Verification items for the finished model (mm, model axes). A direction names the side the tool comes from. Coordinates: 2 decimals unless noted, no trailing zeros. Order: outer loops, then holes, each group sorted by start corner. A loop starts at its lowest first (then second) coordinate and runs counter-clockwise, first axis right, second up. Notation, with made-up numbers: M 27,64 L 43,64 A22 cw 43,103 Z; hole C 62,48 d11. An arc over 180 degrees is marked long. Return JSON: item names as keys, results as strings.
Autodesk Inventor part; units mm, degrees
ref_plane "YZ Plane" through (0, 0, 0) normal (1, 0, 0) x (0, 1, 0)
ref_plane "XZ Plane" through (0, 0, 0) normal (0, 1, 0) x (-1, 0, 0)
ref_plane "XY Plane" through (0, 0, 0) normal (0, 0, 1) x (1, 0, 0)
sketch "Esquisse1" plane through (0, 0, 0) normal (0, 1, 0) x (-1, 0, 0)
  circle A0 centre (0, 0) radius 1.45
  circle A1 centre (0, 0) radius 4
  dimension "d0" = 8
  dimension "d1" = 2.9
extrude "Extrusion1" add sketch "Esquisse1" along normal blind 7
sketch "Esquisse2" plane through (0, 7, 0) normal (0, 1, 0) x (1, 0, 0)
  circle A0 centre (0, 0) radius 1.45
  circle A1 centre (0, 0) radius 4
  arc A2 (-2.3049, 1.5) -> (2.3049, 1.5) centre (0, 0) ccw
  line L0 (-2.3049, 1.5) -> (2.3049, 1.5)
  arc A3 (2.3049, 1.5) -> (-2.3049, 1.5) centre (0, 0) ccw construction
  dimension "d4" = 5.5
  dimension "d5" = 1.5
extrude "Extrusion2" add sketch "Esquisse2" along normal blind 8 contours A1
sketch "Esquisse3" plane through (-2.3049, 7, -1.5) normal (0, 0, 1) x (1, 0, 0)
  line L0 (4.6098, 0) -> (0, 0)
  line L1 (4.6098, 0) -> (4.6098, 8)
  line L2 (0, 8) -> (4.6098, 8)
  line L3 (1.3049, 7.2) -> (3.3049, 7.2)
  line L4 (3.3049, 7.2) -> (3.3049, 0.8)
  line L5 (3.3049, 0.8) -> (1.3049, 0.8)
  line L6 (1.3049, 0.8) -> (1.3049, 7.2)
  point P0 (2.3049, -7)
  dimension "d8" = 2
  dimension "d9" = 0.8
  dimension "d10" = 0.8
  dimension "d11" = 1.3049
  dimension "d12" = 4.6098
extrude "Extrusion3" cut sketch "Esquisse3" along normal through all both and the other way through all
equation "\"d9\" = d10"
equation "\"d11\" = -0.5 * d8 + 0.5 * d12"
properties part number "axe"
Q1. Cross-section at C-C, the plane y = 6.75. Record the boundary of the cut face in (x, z), and give its area (3 significant figures).
Values:
{"outline": "C 0,0 d8; hole C 0,0 d2.9", "area": "43.7 mm^2"}
Q2. Material ranges on line 1 along X through (y, z) = (11, 0); line 2 along Z through (x, y) = (0, 3.75); line 3 along Y through (x, z) = (0, 3), recorded low to high.
Values:
{"line 1": "-4 to -2.75, 2.75 to 4", "line 2": "-4 to -1.45, 1.45 to 4", "line 3": "0 to 7.8, 14.2 to 15"}
Q3. Tool access check on faces 5 (the face through (-2, 11, -1.5)), 6 (the face through (0, 7, 4)), 7 (the face through (0, 7.8, 3)). Record the directions out of +Z, -Z, +X, -X, +Y, -Y that give a thin tool (end or side, any length) a straight path to the whole face; none if there is none.
Values:
{"face 5": "+Y", "face 6": "+Y, -Y", "face 7": "+Z, -Z"}
Q4. Go/stop test with flat-tipped pins: pin 1 (2.5 mm diameter, centred on x = 0, z = 0, fed in from -Y); pin 2 (4 mm diameter, centred on y = 4, z = 2.5, fed in from +X); pin 3 (2.5 mm diameter, centred on x = 0.5, y = 12.5, fed in from +Z); pin 4 (3 mm diameter, centred on y = 8, z = 3, fed in from -X). Record where each tip stops, or that it passes through.
Values:
{"pin 1": "through", "pin 2": "x = 3.97", "pin 3": "z = 3.87", "pin 4": "x = -3.71"}
Q5. Draft check along Y on faces 1 (the face through (1.45, 3.45, -0.06)), 2 (the face through (0, 14.2, 3)), 3 (the face through (-2, 0, 0)), 4 (the face through (0, 15, -2)). Enter one of: pulls with the +Y half, pulls with the -Y half, needs draft (parallel to the pull), parting line crosses it, or undercut.
Values:
{"face 1": "needs draft", "face 2": "undercut", "face 3": "pulls with the -Y half", "face 4": "pulls with the +Y half"}
Q6. Cross-section at A-A, the plane y = 9. Record the boundary of the cut face in (x, z).
Values:
{"outline": "M -2.3,-1.5 A2.75 cw -1,2.56 L -1,3.87 A4 ccw -1,-3.87 L -1,-1.5 Z; M 1,-3.87 A4 ccw 1,3.87 L 1,2.56 A2.75 cw 2.3,-1.5 L 1,-1.5 Z"}
